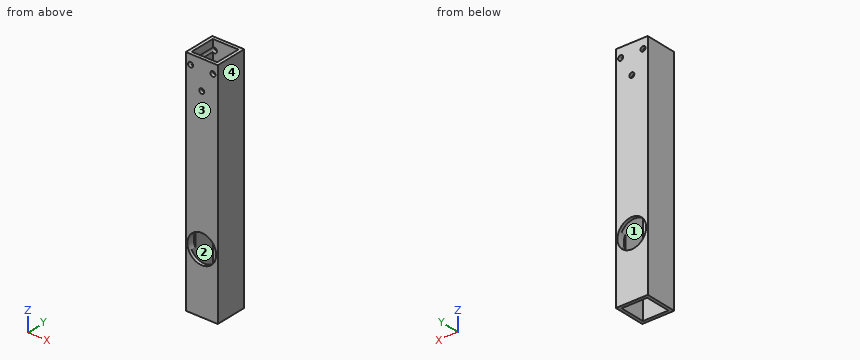
```python
from build123d import *

# Parameters (mm, degrees)
BOSS_EXTRUDE1_DEPTH      = 114.3
BOSS_EXTRUDE1_DEPTH_BACK = 114.3
SKETCH3_W                = 31.75
SKETCH3_H                = 31.75
SKETCH3_W_2              = 25.4
SKETCH3_H_2              = 25.4
F_10_CLEARANCE_HOLE1_D   = 4.9784
SKETCH7_R                = 14.2875
CUT_EXTRUDE1_DEPTH       = 7.62
CUT_EXTRUDE2_START       = -7.62
SKETCH8_R                = 14.2875
CUT_EXTRUDE2_DEPTH       = 7.62


with BuildPart() as part:
    # Sketch3 → Boss-Extrude1 (new, two sides: drawn at the far end of the back side and taken through both)
    with BuildSketch(Plane.XY.offset(-BOSS_EXTRUDE1_DEPTH_BACK)):
        Rectangle(SKETCH3_W, SKETCH3_H)
        Rectangle(SKETCH3_W_2, SKETCH3_H_2, mode=Mode.SUBTRACT)
    extrude(amount=BOSS_EXTRUDE1_DEPTH + BOSS_EXTRUDE1_DEPTH_BACK)

    # #10 Clearance Hole1 (through all)
    with Locations(Plane(origin=(0, 15.875, 0), x_dir=(1, 0, 0), z_dir=(0, 1, 0))):
        with Locations((-11.1125, -104.775), (11.1125, -104.775), (0, -85.5472)):
            Hole(F_10_CLEARANCE_HOLE1_D / 2)

    # Sketch7 → Cut-Extrude1 (cut)
    with BuildSketch(Plane(origin=(0, 15.875, 0), x_dir=(1, 0, 0), z_dir=(0, 1, 0))):
        with Locations(Location((0, 53.975, 0), (0, 0, 270))):
            Circle(SKETCH7_R)
    extrude(amount=-CUT_EXTRUDE1_DEPTH, mode=Mode.SUBTRACT)

    # Sketch8 → Cut-Extrude2 (cut)
    with BuildSketch(Plane.XZ.offset(15.875).offset(CUT_EXTRUDE2_START)):
        with Locations(Location((0, -53.975, 0), (0, 0, 90))):
            Circle(SKETCH8_R)
    extrude(amount=CUT_EXTRUDE2_DEPTH, mode=Mode.SUBTRACT)


solid = part.part
```
Verification items for the finished model (mm, model axes). Face numbers are marked on the shaded views. Round coordinates to 2 decimals unless told otherwise and drop trailing zeros. Order: outer loops, then holes, each group sorted by start corner. A loop starts at its lowest first (then second) coordinate and runs counter-clockwise, first axis right, second up. Notation, with made-up numbers: (4.25, 46.25) - (47.25, 46.25) arc R25 cw to (47.25, 69.25) - close; hole circle Ø5 at (-18, 82.25). An arc over 180 degrees is marked (long way). Use CSV: the item, a comma, the result in double quotes. Start each with the question number.
1) Section check A-A, the plane x = 0. Record the cut outline in (y, z) (1 decimal).
2) Go/stop test with flat-tipped pins: P1, Ø10, axis at x = -2, z = -59, coming from the +Y side; P2, Ø1.3, axis at x = -13, z = -56.5, coming from the +Y side (3 decimals); P3, Ø0.8, axis at x = -13.5, z = -54.5, coming from the -Y side (3 decimals). Record where each tip stops, or that it passes through.
3) Thickness scan on L1, parallel to Z at x = 0, y = 13.5; L2, parallel to X at y = -11, z = -88.5 (3 decimals). Record the ranges inside material, lowest first.
4) Section check D-D, the plane x = -10.5. Record the cut outline in (y, z) (3 decimals).
5) Mould release check, pull along X, two halves, no side actions. Record for the marked faces 1, 2, 3 and 4: +X half, -X half, draft (parallel to the pull), parting line (faces both ways), or undercut.
6) Section check B-B, the plane y = -3. Record the cut outline in (x, z) (1 decimal), plus the area to 3 significant figures.
7) Section check C-C, the plane z = -33. Record the cut outline in (x, y) (3 decimals), plus the area to 3 significant figures.
Answers:
1,outline,"(-15.9, -114.3) - (-12.7, -114.3) - (-12.7, -68.3) - (-15.9, -68.3) - close; (-15.9, -39.7) - (-12.7, -39.7) - (-12.7, 83.1) - (-15.9, 83.1) - close; (-15.9, 88) - (-12.7, 88) - (-12.7, 114.3) - (-15.9, 114.3) - close; (12.7, -114.3) - (15.9, -114.3) - (15.9, -68.3) - (12.7, -68.3) - close; (12.7, -39.7) - (15.9, -39.7) - (15.9, 83.1) - (12.7, 83.1) - close; (12.7, 88) - (15.9, 88) - (15.9, 114.3) - (12.7, 114.3) - close"
2,P1,"passes through"
2,P2,"stops at y = 8.255"
2,P3,"stops at y = -8.255"
3,L1,"z = -114.3 to -68.26, -39.69 to 83.06, 88.04 to 114.3"
3,L2,"x = -15.875 to -12.7, 12.7 to 15.875"
4,outline,"(-15.875, -114.3) - (-12.7, -114.3) - (-12.7, -63.664) - (-15.875, -63.664) - close; (-15.875, -44.286) - (-12.7, -44.286) - (-12.7, 102.362) - (-15.875, 102.362) - close; (-15.875, 107.188) - (-12.7, 107.188) - (-12.7, 114.3) - (-15.875, 114.3) - close; (12.7, -114.3) - (15.875, -114.3) - (15.875, -63.664) - (12.7, -63.664) - close; (12.7, -44.286) - (15.875, -44.286) - (15.875, 102.362) - (12.7, 102.362) - close; (12.7, 107.188) - (15.875, 107.188) - (15.875, 114.3) - (12.7, 114.3) - close"
5,face 1,"undercut"
5,face 2,"undercut"
5,face 3,"draft"
5,face 4,"+X half"
6,outline,"(-15.9, -114.3) - (-12.7, -114.3) - (-12.7, 102.9) arc R2.5 cw to (-12.7, 106.7) - (-12.7, 114.3) - (-15.9, 114.3) - close; (12.7, -114.3) - (15.9, -114.3) - (15.9, 114.3) - (12.7, 114.3) - (12.7, 106.7) arc R2.5 cw to (12.7, 102.9) - close"
6,area,"1,450 mm²"
7,outline,"(-15.875, -15.875) - (15.875, -15.875) - (15.875, 15.875) - (-15.875, 15.875) - close; hole (-12.7, -12.7) - (12.7, -12.7) - (12.7, 12.7) - (-12.7, 12.7) - close"
7,area,"363 mm²"
